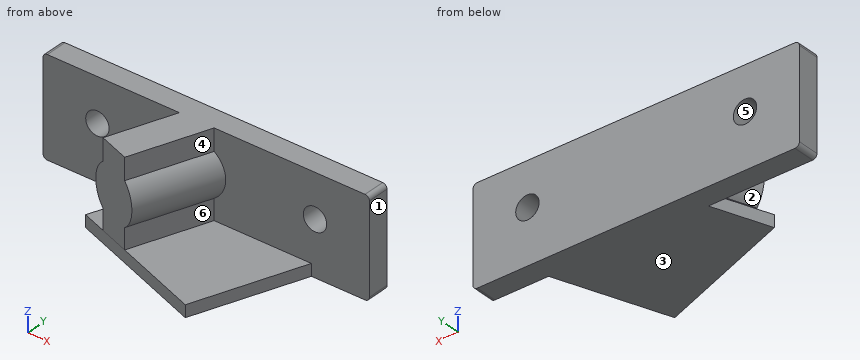
```python
from build123d import *

# Parameters (mm, degrees)
SKETCH_1_W      = 60
SKETCH_1_H      = 18
SKETCH_1_R      = 2.15
EXTRUDE_1_DEPTH = 4
EXTRUDE_3_DEPTH = 2.2
FILLET_1_R      = 0.8
EXTRUDE_4_DEPTH = 15.801607137


with BuildPart() as part:
    # 草图1 → 凸台-拉伸1 (new body)
    with BuildSketch(Plane(origin=(0, 0, 0), x_dir=(1, 0, 0), z_dir=(0, 1, 0))):
        with Locations((0, 9)):
            Rectangle(SKETCH_1_W, SKETCH_1_H)
        with Locations(Location((-20, 8, 0), (0, 0, 270))):
            Circle(SKETCH_1_R, mode=Mode.SUBTRACT)
        with Locations(Location((20, 8, 0), (0, 0, 270))):
            Circle(SKETCH_1_R, mode=Mode.SUBTRACT)
    extrude(amount=EXTRUDE_1_DEPTH)

    # 草图5 → 凸台-拉伸3 (add)
    with BuildSketch(Plane(origin=(0, 0, -18), x_dir=(-1, 0, 0), z_dir=(0, 0, -1))):
        Polygon((-19.332346445, 0), (10.038960076, 0), (13.801181652, -10.336618829), (-12.134334681, -19.776374784), align=None)
    extrude(amount=-EXTRUDE_3_DEPTH)

    # 圆角1
    fillet_1_edges = [part.edges().sort_by_distance(p)[0] for p in [
        (-30, 2, -18),
        (30, 2, -18),
        (30, 2, 0),
        (-30, 2, 0),
    ]]
    fillet(fillet_1_edges, radius=FILLET_1_R)

    # 草图4 → 凸台-拉伸4 (add)
    with BuildSketch(Plane(origin=(0.467911114, 1.285575219, 0), x_dir=(0, 0, -1), z_dir=(0.34202014332566943, 0.9396926207859081, 0))):
        with BuildLine():
            Line((0, 4.633536704), (4, 4.633536704))
            ThreePointArc((4, 4.633536704), (8, 6.633536704), (12, 4.633536704))
            Line((12, 4.633536704), (18, 4.633536704))
            Line((18, 4.633536704), (18, -1.366463296))
            Line((18, -1.366463296), (12, -1.366463296))
            ThreePointArc((12, -1.366463296), (8, -3.366463296), (4, -1.366463296))
            Line((4, -1.366463296), (0, -1.366463296))
            Line((0, -1.366463296), (0, 4.633536704))
        make_face()
    extrude(amount=-EXTRUDE_4_DEPTH)


solid = part.part
```
The listing builds one solid part. Answer for the finished solid, in the listing's coordinates (mm). Face numbers are marked on the shaded views. A direction names the side the tool comes from. Give positions to 0.01 mm unless a question says otherwise; leave off trailing zeros. Order: outer loops, then holes, each group sorted by start corner. A loop starts at its lowest first (then second) coordinate and runs counter-clockwise, first axis right, second up.
1) Find section C-C on z = -8. Write down the section's boundary in (x, y).
Reported:
outline: (-30, 0) - (-22.15, 0) - (-22.15, 4) - (-30, 4) - close; (-17.85, 0) - (-7.06, 0) - (-11.17, -11.29) - (-1.77, -14.71) - (3.58, 0) - (17.85, 0) - (17.85, 4) - (-17.85, 4) - close; (22.15, 0) - (30, 0) - (30, 4) - (22.15, 4) - close
2) Determine the mould class of the marked faces 1, 2 and 3 for opening direction Z: pulls with the +Z half, pulls with the -Z half, needs draft (parallel to the pull), parting line crosses it, or undercut.
Reported:
face 1: needs draft
face 2: undercut
face 3: pulls with the -Z half
3) Given P1, Ø10, axis at x = -10.5, y = -13, coming from the +Z side; P2, Ø7, axis at x = -20, z = -8, coming from the -Y side; P3, Ø8, axis at x = -8, z = -9.5, coming from the -Y side; P4, Ø5, axis at y = -6.5, z = -16, coming from the -X side, each flat-ended and moving along its own axis, determine where each tip first touches the part or whether it passes through.
Reported:
P1: stops at z = 0
P2: stops at y = 0
P3: stops at y = -13.9
P4: stops at x = -13.31
4) Find section A-A on x = 21. Write down the section's boundary in (y, z), then the cut area to 3 significant figures.
Reported:
outline: (0, -18) - (4, -18) - (4, -9.9) - (0, -9.9) - close; (0, -6.1) - (4, -6.1) - (4, 0) - (0, 0) - close
area: 56.8 mm2
5) Find section D-D on x = 9. Write down the section's boundary in (y, z).
Reported:
outline: (-18.64, -18) - (4, -18) - (4, 0) - (0, 0) - (0, -15.8) - (-18.64, -15.8) - close
6) For the marked faces 4, 5 and 6, determine the directions among +Z, -Z, +X, -X, +Y, -Y from which every point of the face is accessible in a straight line to the end or side of a thin tool.
Reported:
face 4: +Z, +X, -Y
face 5: +Y, -Y
face 6: +X, -Y
7) Find section B-B on z = -16.5. Write down the section's boundary in (x, y), then the cut area to 3 significant figures.
Reported:
outline: (-30, 0) - (-10.04, 0) - (-13.8, -10.34) - (12.13, -19.78) - (19.33, 0) - (30, 0) - (30, 4) - (-30, 4) - close
area: 682 mm2
8) Consider line 1 along X through (y, z) = (0.8, -8); line 2 along Y through (x, z) = (14.5, -11.5); line 3 along X through (y, z) = (1, -0.75). Determine where each line is inside the solid, lowest interval first.
Reported:
line 1: x = -30 to -22.15, -17.85 to 17.85, 22.15 to 30
line 2: y = 0 to 4
line 3: x = -30 to 30
